Here's the drawing with two shaded views (mm, measured from the low corner). I have some questions. Round coordinates to 2 decimals unless told otherwise and drop trailing zeros. Order: outer loops, then holes, each group sorted by start corner. A loop starts at its lowest first (then second) coordinate and runs counter-clockwise, first axis right, second up. Notation, with made-up numbers: (58, 86.5) - (69, 86.5) arc R23 cw to (69, 96.5) - close; hole circle Ø4 at (12.25, -39.5). An arc over 180 degrees is marked (long way). One line per item, written item: value.
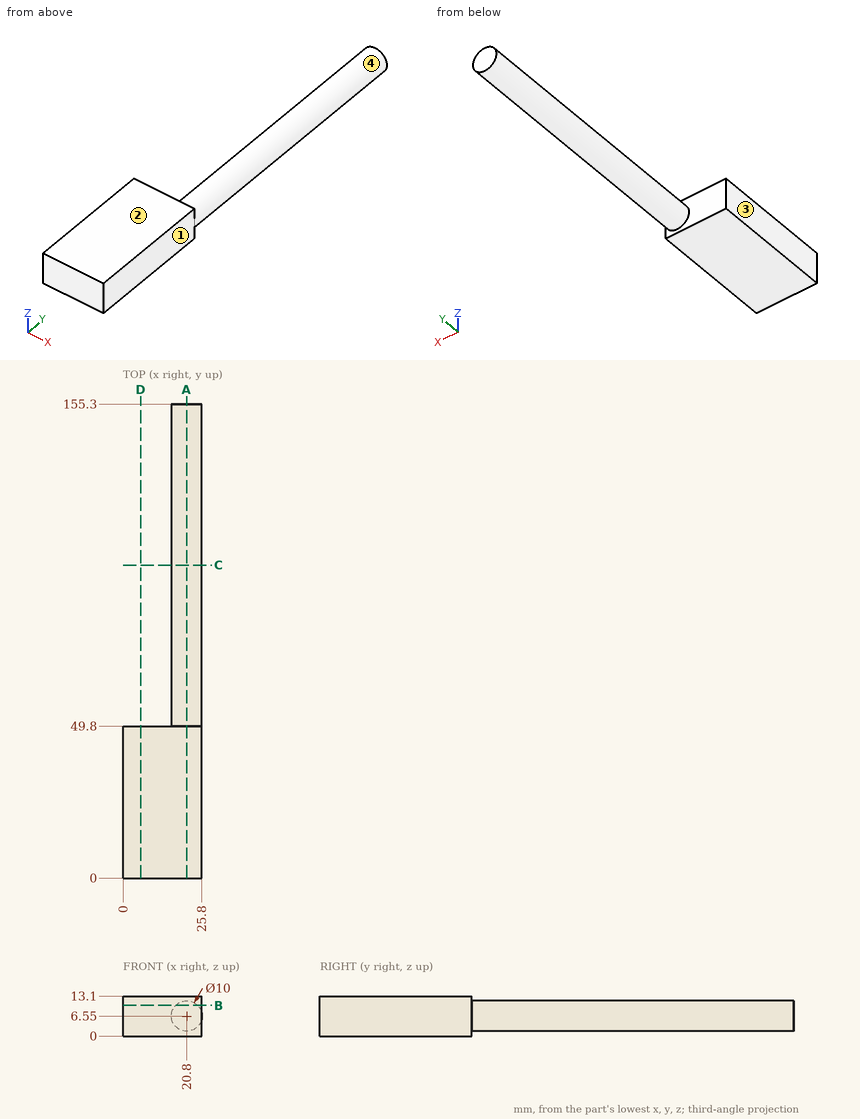
Q1. If we section it at D-D, the plane x = 5.75: Please give me the cut outline in (y, z), then the cut area to 3 significant figures.
Results list:
outline: (0, 0) - (49.8, 0) - (49.8, 13.1) - (0, 13.1) - close
area: 652 mm²
Q2. If we section it at A-A, the plane x = 20.8: Please give me the cut outline in (y, z), then the cut area to 3 significant figures.
Results list:
outline: (0, 0) - (49.8, 0) - (49.8, 1.55) - (155.3, 1.55) - (155.3, 11.55) - (49.8, 11.55) - (49.8, 13.1) - (0, 13.1) - close
area: 1,710 mm²
Q3. We'd pull the mould along X, two halves only. Please class the marked faces 1, 2, 3 and 4: released by +X, released by -X, zero draft, split by the parting line, or undercut.
Results list:
face 1: released by +X
face 2: zero draft
face 3: released by -X
face 4: split by the parting line
Q4. If I drill on line 1 along Y through (x, z) = (16, 10.5); line 2 along X through (y, z) = (108.5, 6.75); line 3 along Z through (x, y) = (16.25, 111), over which ranges is the centre line in solid material (lowest first)?
Results list:
line 1: 0 to 49.8
line 2: 15.8 to 25.8
line 3: 4.48 to 8.62
Q5. Will these pins go through, and if not, where does the flat tip stop? pin 1 (2 mm diameter, centred on x = 19, y = 125, fed in from +Z); pin 2 (1 mm diameter, centred on y = 50.5, z = 11.5, fed in from -X); pin 3 (2 mm diameter, centred on y = 132, z = 8, fed in from -X); pin 4 (2 mm diameter, centred on x = 6, y = 52, fed in from -Z).
Results list:
pin 1: z = 11.49
pin 2: x = 18.52
pin 3: x = 15.82
pin 4: through
Q6. If we section it at B-B, the plane z = 10: Please give me the cut outline in (x, y), then the cut area to 3 significant figures.
Results list:
outline: (0, 0) - (25.8, 0) - (25.8, 49.8) - (24.42, 49.8) - (24.42, 155.3) - (17.18, 155.3) - (17.18, 49.8) - (0, 49.8) - close
area: 2,050 mm²
Q7. If we section it at C-C, the plane y = 102.5: Please give me the cut outline in (x, z).
Results list:
outline: circle Ø10 at (20.8, 6.55)
